Model file for the job. Use its own axes, mm. A direction names the side the tool comes from. Round coordinates to 2 decimals unless told otherwise and drop trailing zeros. Loops run counter-clockwise (first coordinate to the right, second up) from the corner with the lowest first, then second, coordinate; pieces in that order, holes last. Notation, with made-up numbers: (69, 1.5) -> (79, 1.5) arc R12 cw to (79, 14.5) -> close; hole circle Ø9 at (-34.5, 22). An arc over 180 degrees is marked (long way). Use a Markdown table: item, result.
from build123d import *

# Parameters (mm, degrees)
BRIDA_BASE1_DEPTH     = 19.5
CROQUIS9_R            = 1.5
CORTAR_EXTRUIR4_DEPTH = 0.5
CROQUIS10_R           = 1.5
CORTAR_EXTRUIR5_DEPTH = 0.5
CROQUIS8_R            = 1.5
CORTAR_EXTRUIR3_DEPTH = 10


# Sheet-metal steps are written as plain solids
with BuildPart() as part:
    # Croquis1 → Brida base1 (new body)
    with BuildSketch(Plane(origin=(0, 0, 0), x_dir=(0, 0, -1), z_dir=(1, 0, 0))):
        with BuildLine():
            Line((-8.25, 24.950879865), (-0.5, 24.950879865))
            ThreePointArc((-0.5, 24.950879865), (-0.146446609, 24.804433255), (0, 24.450879865))
            Line((0, 24.450879865), (0, 8.950879865))
            Line((0, 8.950879865), (0.5, 8.950879865))
            Line((0.5, 8.950879865), (0.5, 24.450879865))
            ThreePointArc((0.5, 24.450879865), (0.207106781, 25.157986646), (-0.5, 25.450879865))
            Line((-0.5, 25.450879865), (-8.25, 25.450879865))
            Line((-8.25, 25.450879865), (-8.25, 24.950879865))
        make_face()
    extrude(amount=BRIDA_BASE1_DEPTH)

    # Croquis9 → Cortar-Extruir4 (cut)
    with BuildSketch(Plane(origin=(0, 0, -0.5), x_dir=(-1, 0, 0), z_dir=(0, 0, -1))):
        with BuildLine():
            ThreePointArc((-6.25, 17.200879865), (-9.75, 20.700879865), (-13.25, 17.200879865))
            Line((-13.25, 17.200879865), (-13.25, 8.950879865))
            Line((-13.25, 8.950879865), (-6.25, 8.950879865))
            Line((-6.25, 8.950879865), (-6.25, 17.200879865))
        make_face()
        with Locations(Location((-15.21, 17.200879865, 0), (0, 0, 90))):
            Circle(CROQUIS9_R)
        with Locations(Location((-4.29, 17.200879865, 0), (0, 0, 90))):
            Circle(CROQUIS9_R)
    extrude(amount=-CORTAR_EXTRUIR4_DEPTH, mode=Mode.SUBTRACT)

    # Croquis10 → Cortar-Extruir5 (cut)
    with BuildSketch(Plane(origin=(0, 25.450879865, 0), x_dir=(1, 0, 0), z_dir=(0, 1, 0))):
        with Locations(Location((9.75, -4.375, 0), (0, 0, 270))):
            Circle(CROQUIS10_R)
    extrude(amount=-CORTAR_EXTRUIR5_DEPTH, mode=Mode.SUBTRACT)

    # Croquis8 → Cortar-Extruir3 (cut)
    with BuildSketch(Plane(origin=(0, 25.450879865, 0), x_dir=(1, 0, 0), z_dir=(0, 1, 0))):
        with Locations((9.75, -4.125)):
            Circle(CROQUIS8_R)
    extrude(amount=-CORTAR_EXTRUIR3_DEPTH, mode=Mode.SUBTRACT)


solid = part.part
Q1. Flat gauge pins, fed straight in: pin 1 (4.5 mm diameter, centred on x = 6, y = 13.5, fed in from +Z); pin 2 (4 mm diameter, centred on x = 5.5, z = 4, fed in from -Y). Where does each tip first touch, or does it go through?
Results list:
| item | result |
|---|---|
| pin 1 | stops at z = 0 |
| pin 2 | stops at y = 24.95 |
Q2. Band-saw the part on A-A, the plane x = 9.75. Give the cut face in (y, z) (3 decimals).
Results list:
| item | result |
|---|---|
| outline | (20.701, -0.5) -> (24.451, -0.5) arc R1 ccw to (25.451, 0.5) -> (25.451, 2.625) -> (24.951, 2.625) -> (24.951, 0.5) arc R0.5 cw to (24.451, 0) -> (20.701, 0) -> close; (24.951, 5.875) -> (25.451, 5.875) -> (25.451, 8.25) -> (24.951, 8.25) -> close |
Q3. Band-saw the part on D-D, the plane z = 5.5. Give the cut face in (x, y).
Results list:
| item | result |
|---|---|
| outline | (0, 24.95) -> (8.76, 24.95) -> (8.76, 25.45) -> (0, 25.45) -> close; (10.74, 24.95) -> (19.5, 24.95) -> (19.5, 25.45) -> (10.74, 25.45) -> close |
Q4. Pull direction Y, two halves, no side cores. Call faces 4 (the face through (9.715, 25.204, 5.875)), 5 (the face through (4.356, 15.702, -0.254)), 6 (the face through (9.614, 25.15, -0.215)): released by +Y, released by -Y, zero draft, split by the parting line, or undercut.
Results list:
| item | result |
|---|---|
| face 4 | zero draft |
| face 5 | undercut |
| face 6 | released by +Y |
Q5. Band-saw the part on C-C, the plane x = 15.21. Give the cut face in (y, z), plus the area to 3 significant figures.
Results list:
| item | result |
|---|---|
| outline | (8.95, -0.5) -> (15.7, -0.5) -> (15.7, 0) -> (8.95, 0) -> close; (18.7, -0.5) -> (24.45, -0.5) arc R1 ccw to (25.45, 0.5) -> (25.45, 8.25) -> (24.95, 8.25) -> (24.95, 0.5) arc R0.5 cw to (24.45, 0) -> (18.7, 0) -> close |
| area | 10.7 mm² |
Q6. Tool access for faces 1 (the face through (11.8, 20.3, 0)), 2 (the face through (0, 20.9, -0.3)), 3 (the face through (9.785, 25.204, 2.625)): list every direction of +Z, -Z, +X, -X, +Y, -Y with a clear straight run to the whole face (end or side of a thin tool).
Results list:
| item | result |
|---|---|
| face 1 | +Z, +X, -X, -Y |
| face 2 | +Z, -Z, -X, +Y, -Y |
| face 3 | +Y, -Y |
Q7. Drill centre lines: L1, parallel to Y at x = 11.25, z = 7.5; L2, parallel to Z at x = 15.75, y = 15.5; L3, parallel to Z at x = 9.75, y = 25.1 (3 decimals). Where is each one in solid material? Low to high. Write a range as from..to.
Results list:
| item | result |
|---|---|
| L1 | y = 24.95..25.45 |
| L2 | z = -0.5..0 |
| L3 | z = -0.261..2.625, 5.875..8.25 |
Q8. Band-saw the part on B-B, the plane z = 4. Give the cut face in (x, y).
Results list:
| item | result |
|---|---|
| outline | (0, 24.95) -> (8.26, 24.95) -> (8.26, 25.45) -> (0, 25.45) -> close; (11.24, 24.95) -> (19.5, 24.95) -> (19.5, 25.45) -> (11.24, 25.45) -> close |
